Part model, mm, in its own coordinate system. A direction names the side the tool comes from. Coordinates: 2 decimals unless noted, no trailing zeros. Order: outer loops, then holes, each group sorted by start corner. A loop starts at its lowest first (then second) coordinate and runs counter-clockwise, first axis right, second up. Notation, with made-up numbers: M 49.25,-35 L 105.25,-35 A18 ccw 105.25,-2 Z; hole C 82,68 d1. An arc over 180 degrees is marked long. Write item = value, one per line. Start each with the question number.
from build123d import *

# Parameters (mm, degrees)
SKETCH1_R           = 3.81
BOSS_EXTRUDE2_DEPTH = 10.16
BOSS_EXTRUDE3_DEPTH = 5.08
SKETCH5_R           = 2.413
CUT_EXTRUDE1_DEPTH  = 5.08


with BuildPart() as part:
    # Sketch1 → Boss-Extrude2 (new body)
    with BuildSketch(Plane.XY):
        Circle(SKETCH1_R)
    extrude(amount=BOSS_EXTRUDE2_DEPTH)

    # Sketch4 → Boss-Extrude3 (add)
    with BuildSketch(Plane.XY.offset(10.16)):
        Polygon((-2.032318753, 3.222697703), (2.032318753, 3.222697703), (0, 36.83), align=None)
    extrude(amount=-BOSS_EXTRUDE3_DEPTH)

    # Sketch5 → Cut-Extrude1 (cut)
    with BuildSketch(Plane(origin=(0, 0, 0), x_dir=(-1, 0, 0), z_dir=(0, 0, -1))):
        Circle(SKETCH5_R)
    extrude(amount=-CUT_EXTRUDE1_DEPTH, mode=Mode.SUBTRACT)


solid = part.part
Item 1: Flat gauge pins, fed straight in: pin 1 (3 mm diameter, centred on x = 0.5, z = 1.5, fed in from +Y); pin 2 (4.5 mm diameter, centred on x = 1, y = 13.5, fed in from -Z); pin 3 (1.5 mm diameter, centred on x = -2, y = 14, fed in from +Z). Where does each tip first touch, or does it go through?
Item 2: Cut at D-D, the plane z = 7. Write the cut outline in (x, y).
Item 3: 3-axis set-ups, long thin cutter, end or side, ignore diameter. For faces 1 (the flat face through (0.8, -2.5, 0)), 2 (the flat face through (0, 0, 5.08)): which of +Z, -Z, +X, -X, +Y, -Y reach the whole face in a straight line?
Item 4: Cut at B-B, the plane z = 4.5. Write the cut outline in (x, y), and give its area (3 significant figures).
Item 5: Wall check: line 1 along Y through (x, z) = (0, 1.6); line 2 along Z through (x, y) = (-0.25, 28); line 3 along X through (y, z) = (4, 7). Give the ranges that are in metal, low to high. Write a range as [from, to].
Item 6: Cut at A-A, the plane y = 0. Write the cut outline in (x, z).
Item 7: Pull direction X, two halves, no side cores. Call faces 3 (the cylindrical face through (1.915, -1.468, 2.504)), 4 (the flat face through (0, 8, 10.16)), 5 (the flat face through (-1, 20.3, 7.7)), 6 (the flat face through (1.03, 19.79, 7.66)): pulls with the +X half, pulls with the -X half, needs draft (parallel to the pull), parting line crosses it, or undercut.
Item 8: Cut at C-C, the plane x = -1.5. Write the cut outline in (y, z).
Filled sheet:
q1.pin_1 = 3.81
q1.pin_2 = 5.08
q1.pin_3 = 10.16
q2.outline = M -2.03,3.22 A3.81 ccw long 2.03,3.22 L 0,36.83 Z
q3.face_1 = -Z, +X, -X, +Y, -Y
q3.face_2 = -Z
q4.outline = C 0,0 d7.62; hole C 0,0 d4.83
q4.area = 27.3 mm2
q5.line_1 = [-3.81, -2.41], [2.41, 3.81]
q5.line_2 = [5.08, 10.16]
q5.line_3 = [-1.99, 1.99]
q6.outline = M -3.81,0 L -2.41,0 L -2.41,5.08 L 2.41,5.08 L 2.41,0 L 3.81,0 L 3.81,10.16 L -3.81,10.16 Z
q7.face_3 = undercut
q7.face_4 = needs draft
q7.face_5 = pulls with the -X half
q7.face_6 = pulls with the +X half
q8.outline = M -3.5,0 L -1.89,0 L -1.89,5.08 L 1.89,5.08 L 1.89,0 L 3.5,0 L 3.5,5.08 L 12.03,5.08 L 12.03,10.16 L -3.5,10.16 Z
